Read the model definition and answer for the solid it produces. Units are mm, in the model's axes. Face numbers are marked on the shaded views. Give positions to 0.01 mm unless a question says otherwise; leave off trailing zeros. Loops run counter-clockwise (first coordinate to the right, second up) from the corner with the lowest first, then second, coordinate; pieces in that order, holes last. Notation, with made-up numbers: (21.25, 27) - (70.25, 27) arc R19 cw to (70.25, 36) - close; hole circle Ø5 at (53.5, -29.5). An arc over 180 degrees is marked (long way). Write item = value, one per line. Start each with the question number.
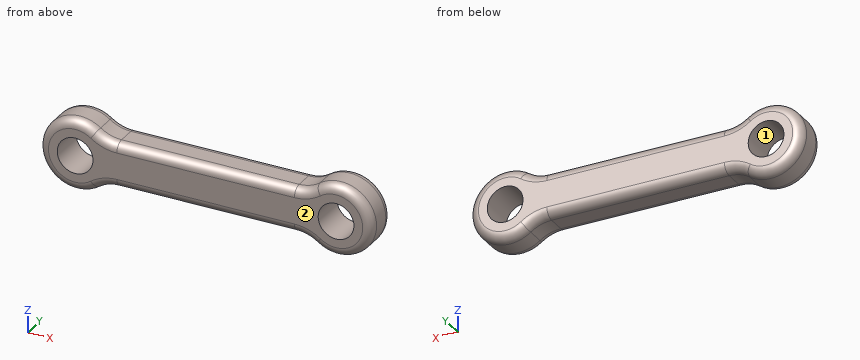
from build123d import *

# Parameters (mm, degrees)
SKETCH1_R           = 5
BOSS_EXTRUDE1_DEPTH = 10
FILLET1_R           = 2.54


with BuildPart() as part:
    # Sketch1 → Boss-Extrude1 (new body)
    with BuildSketch(Plane(origin=(0, 0, 0), x_dir=(1, 0, 0), z_dir=(0, 1, 0))):
        with BuildLine():
            Line((-6.590776184, -6.25), (43.090776184, -6.25))
            ThreePointArc((43.090776184, -6.25), (46.152638362, -6.730283618), (48.920388092, -8.125))
            ThreePointArc((48.920388092, -8.125), (64.75, 0), (48.920388092, 8.125))
            ThreePointArc((48.920388092, 8.125), (46.152638362, 6.730283618), (43.090776184, 6.25))
            Line((43.090776184, 6.25), (-6.590776184, 6.25))
            ThreePointArc((-6.590776184, 6.25), (-9.652638362, 6.730283618), (-12.420388092, 8.125))
            ThreePointArc((-12.420388092, 8.125), (-28.25, 0), (-12.420388092, -8.125))
            ThreePointArc((-12.420388092, -8.125), (-9.652638362, -6.730283618), (-6.590776184, -6.25))
        make_face()
        with Locations((-18.25, 0)):
            Circle(SKETCH1_R, mode=Mode.SUBTRACT)
        with Locations((54.75, 0)):
            Circle(SKETCH1_R, mode=Mode.SUBTRACT)
    extrude(amount=BOSS_EXTRUDE1_DEPTH)

    # Fillet1
    fillet1_edges = [part.edges().sort_by_distance(p)[0] for p in [
        (-9.652638362, 10, 6.730283618),
        (-28.25, 0, 0),
        (-9.652638362, 0, -6.730283618),
        (18.25, 10, 6.25),
        (46.152638362, 10, 6.730283618),
        (64.75, 10, 0),
        (46.152638362, 10, -6.730283618),
        (18.25, 10, -6.25),
        (-9.652638362, 10, -6.730283618),
        (-28.25, 10, 0),
        (18.25, 0, -6.25),
        (46.152638362, 0, -6.730283618),
        (64.75, 0, 0),
        (46.152638362, 0, 6.730283618),
        (18.25, 0, 6.25),
        (-9.652638362, 0, 6.730283618),
    ]]
    fillet(fillet1_edges, radius=FILLET1_R)


solid = part.part
1. For a pull along X with two mould halves and no side action, classify the marked faces 1 and 2 as released by +X, released by -X, zero draft, split by the parting line, or undercut.
2. A cutting plane is placed at A-A on y = 3.5. Give the vertices of the cut face in (x, z) (3 decimals), and give its area (3 significant figures).
3. A cutting plane is placed at C-C on z = 0. Give the vertices of the cut face in (x, y).
4. A cutting plane is placed at D-D on y = 8.5. Give the vertices of the cut face in (x, z).
5. Given P1, Ø3, axis at x = -12, y = 1.5, coming from the -Z side; P2, Ø1.5, axis at x = 27.5, y = 4, coming from the -Z side; P3, Ø2, axis at y = 4.5, z = -1.5, coming from the -X side; P4, Ø6, axis at x = 54.75, z = 0, coming from the +Y side, each flat-ended and moving along its own axis, determine where each tip first touches the part or whether it passes through.
6. A cutting plane is placed at B-B on x = -4.5. Give the vertices of the cut face in (y, z), and give its area (3 significant figures).
7. Consider line 1 along X through (y, z) = (7.75, 0); line 2 along Z through (x, y) = (-18.25, 6.5); line 3 along X through (y, z) = (9.75, 3.25). Determine where each line is inside the solid, lowest interval first. Write a range as [from, to].
Reply:
q1.face_1 = undercut
q1.face_2 = zero draft
q2.outline = (-12.42, -8.125) arc R10 cw to (-6.591, -6.25) - (43.091, -6.25) arc R10 cw to (48.92, -8.125) arc R10 ccw (long way) to (48.92, 8.125) arc R10 cw to (43.091, 6.25) - (-6.591, 6.25) arc R10 cw to (-12.42, 8.125) arc R10 ccw (long way) to start; hole circle Ø10 at (-18.25, 0); hole circle Ø10 at (54.75, 0)
q2.area = 1,160 mm^2
q3.outline = (-28.25, 2.54) arc R2.54 ccw to (-25.71, 0) - (-23.25, 0) - (-23.25, 10) - (-25.71, 10) arc R2.54 ccw to (-28.25, 7.46) - close; (-13.25, 0) - (49.75, 0) - (49.75, 10) - (-13.25, 10) - close; (59.75, 0) - (62.21, 0) arc R2.54 ccw to (64.75, 2.54) - (64.75, 7.46) arc R2.54 ccw to (62.21, 10) - (59.75, 10) - close
q4.outline = (-12.55, -7.94) arc R10.22 cw to (-6.59, -6.03) - (43.09, -6.03) arc R10.22 cw to (49.05, -7.94) arc R9.78 ccw (long way) to (49.05, 7.94) arc R10.22 cw to (43.09, 6.03) - (-6.59, 6.03) arc R10.22 cw to (-12.55, 7.94) arc R9.78 ccw (long way) to start; hole circle Ø10 at (-18.25, 0); hole circle Ø10 at (54.75, 0)
q5.P1 = -8.69
q5.P2 = -6.25
q5.P3 = -28.24
q5.P4 = through
q6.outline = (0, -3.71) arc R2.54 ccw to (2.54, -6.25) - (7.46, -6.25) arc R2.54 ccw to (10, -3.71) - (10, 3.71) arc R2.54 ccw to (7.46, 6.25) - (2.54, 6.25) arc R2.54 ccw to (0, 3.71) - close
q6.area = 119 mm^2
q7.line_1 = [-28.23, -23.25], [-13.25, 49.75], [59.75, 64.73]
q7.line_2 = [-10, -5], [5, 10]
q7.line_3 = [-26.17, -22.05], [-14.45, 50.95], [58.55, 62.67]
